Autodesk Inventor part; units mm, degrees
ref_plane "YZ Plane" through (0, 0, 0) normal (1, 0, 0) x (0, 1, 0)
ref_plane "XZ Plane" through (0, 0, 0) normal (0, 1, 0) x (-1, 0, 0)
ref_plane "XY Plane" through (0, 0, 0) normal (0, 0, 1) x (1, 0, 0)
sketch "main" plane through (0, 0, 0) normal (0, 0, 1) x (1, 0, 0)
  circle A0 centre (-9.3272, -22.4282) radius 2.1844
  circle A1 centre (8.5649, -23.9935) radius 2.1844
  circle A2 centre (4.5963, 11.9106) radius 2.1844
  arc A3 (-15.6751, -22.2631) -> (-9.3272, -28.7782) centre (-9.3272, -22.4282) ccw
  arc A4 (8.0027, -30.3186) -> (14.8765, -23.2959) centre (8.5649, -23.9935) ccw
  arc A5 (10.9079, 12.6083) -> (9.0865, 16.4007) centre (4.5963, 11.9106) ccw
  line L0 (-9.3272, -28.7782) -> (8.0027, -30.3186)
  line L1 (10.9079, 12.6083) -> (14.8765, -23.2959)
  circle A6 centre (-8.1037, 24.6106) radius 2.1844
  arc A7 (-3.6135, 29.1007) -> (-14.4515, 24.7757) centre (-8.1037, 24.6106) ccw
  line L2 (9.0865, 16.4007) -> (-3.6135, 29.1007)
  line L3 (-14.4515, 24.7757) -> (-15.6751, -22.2631)
  point P0 (-0.372, -2.6392)
  dimension "d0" = 12.7
  dimension "d1" = 12.7
  dimension "d2" = 12.7
  dimension "d3" = 12.7
sketch "Sketch1" plane through (0, 0, 0) normal (0, 0, 1) x (1, 0, 0)
  circle A0 centre (-1.2236, -47.0388) radius 2.1844
  circle A1 centre (16.6686, -48.6042) radius 2.1844
  circle A2 centre (12.7, -12.7) radius 2.1844
  arc A3 (-7.5714, -46.8737) -> (-1.2236, -53.3888) centre (-1.2236, -47.0388) ccw
  arc A4 (16.1064, -54.9292) -> (22.9802, -47.9065) centre (16.6686, -48.6042) ccw
  arc A5 (19.0116, -12.0024) -> (17.1901, -8.2099) centre (12.7, -12.7) ccw
  line L0 (-1.2236, -53.3888) -> (16.1064, -54.9292)
  line L1 (19.0116, -12.0024) -> (22.9802, -47.9065)
  circle A6 centre (0, 0) radius 2.1844
  arc A7 (4.4901, 4.4901) -> (-6.3479, 0.1651) centre (0, 0) ccw
  line L2 (17.1901, -8.2099) -> (4.4901, 4.4901)
  line L3 (-6.3479, 0.1651) -> (-7.5714, -46.8737)
extrude "Extrusion1" add sketch "Sketch1" along normal blind 1.5875
properties part number "floating-stage-bracket" material "Acetal Resin, Black"
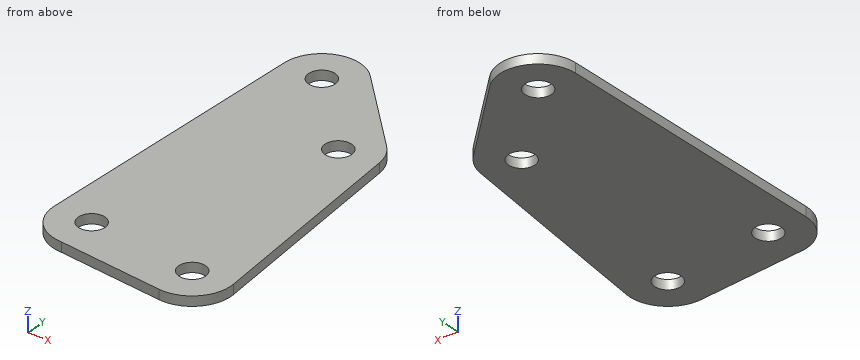
The listing builds one solid part. Answer for the finished solid, in the listing's coordinates (mm). Coordinates: 2 decimals unless noted, no trailing zeros. Loops run counter-clockwise (first coordinate to the right, second up) from the corner with the lowest first, then second, coordinate; pieces in that order, holes last. Notation, with made-up numbers: (47.5, -31.5) - (105.5, -31.5) arc R24 cw to (105.5, -18.5) - close; hole circle Ø7 at (-27, 4). An arc over 180 degrees is marked (long way). Use a Markdown table: item, result. Add a question column.
1) Given pin 1 (4 mm diameter, centred on x = 12.7, y = -12.7, fed in from -Z), flat-ended and moving along its own axis, determine where the tip first touches the part or whether it passes through.
2) The part is cut by section D-D, the plane y = -32. Give the vertices of the cut face in (x, z).
3) The part is cut by section A-A, the plane x = 12.7. Give the vertices of the cut face in (y, z).
4) The part is cut by section C-C, the plane z = 0.65. Give the vertices of the cut face in (x, y).
5) The part is cut by section B-B, the plane x = 0. Give the vertices of the cut face in (y, z), and give its area (3 significant figures).
6) Find the intervals of material crossed by line 1 (X direction, y = -48, z = 0.3); line 2 (Y direction, x = 12.7, z = 0.35); line 3 (Y direction, x = 18, z = 0.1), in increasing order.
Here are the results:
| question | item | result |
|---|---|---|
| 1 | pin 1 | passes through |
| 2 | outline | (-7.18, 0) - (21.22, 0) - (21.22, 1.59) - (-7.18, 1.59) - close |
| 3 | outline | (-54.63, 0) - (-14.88, 0) - (-14.88, 1.59) - (-54.63, 1.59) - close; (-10.52, 0) - (-3.72, 0) - (-3.72, 1.59) - (-10.52, 1.59) - close |
| 4 | outline | (-7.57, -46.87) arc R6.35 ccw to (-1.22, -53.39) - (16.11, -54.93) arc R6.35 ccw to (22.98, -47.91) - (19.01, -12) arc R6.35 ccw to (17.19, -8.21) - (4.49, 4.49) arc R6.35 ccw to (-6.35, 0.17) - close; hole circle Ø4.37 at (-1.22, -47.04); hole circle Ø4.37 at (0, 0); hole circle Ø4.37 at (12.7, -12.7); hole circle Ø4.37 at (16.67, -48.6) |
| 5 | outline | (-53.5, 0) - (-48.85, 0) - (-48.85, 1.59) - (-53.5, 1.59) - close; (-45.23, 0) - (-2.18, 0) - (-2.18, 1.59) - (-45.23, 1.59) - close; (2.18, 0) - (6.35, 0) - (6.35, 1.59) - (2.18, 1.59) - close |
| 5 | area | 82.3 mm^2 |
| 6 | line 1 | x = -7.5 to -3.19, 0.74 to 14.57, 18.77 to 22.99 |
| 6 | line 2 | y = -54.63 to -14.88, -10.52 to -3.72 |
| 6 | line 3 | y = -54.81 to -50.34, -46.87 to -9.2 |
